Geometry check sheet. Reference: the model listing, model coordinates, mm. Give positions to 0.01 mm unless a question says otherwise; leave off trailing zeros. Write each loop counter-clockwise with the first axis right and the second up, starting at its lowest first coordinate (ties: lowest second). Pieces come first, ordered by that corner, then holes.
(1) Thickness scan on line 1 along X through (y, z) = (8.2, 0); line 2 along Z through (x, y) = (21, 7.75); line 3 along Z through (x, y) = (-41.5, 7.5). Record the ranges inside material, lowest first.
(2) Cross-section at B-B (x = 0). Record the boundary of the cut face in (y, z).
(3) Cross-section at A-A (z = 0). Record the boundary of the cut face in (x, y).
(4) Depth check by flat-ended pin: P1, Ø2, axis at x = 12, y = 8.5, coming from the -Z side; P2, Ø5, axis at y = 1, z = -16, coming from the +X side; P3, Ø3, axis at x = 9, y = 2, coming from the -Z side. Enter the tip coordinate at first touch or a pass-through.
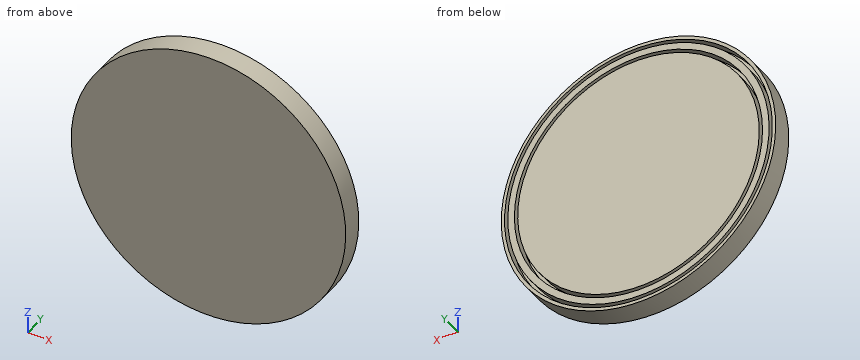
```python
from build123d import *

# Parameters (mm, degrees)
SKETCH2_R           = 62.5
BOSS_EXTRUDE1_DEPTH = 10
SKETCH3_R           = 61
SKETCH3_R_2         = 59.5
SKETCH3_R_3         = 56.5
SKETCH3_R_4         = 55
CUT_EXTRUDE1_DEPTH  = 5


with BuildPart() as part:
    # Sketch2 → Boss-Extrude1 (new body)
    with BuildSketch(Plane(origin=(0, 0, 0), x_dir=(1, 0, 0), z_dir=(0, 1, 0))):
        with Locations(Location((0, 0, 0), (0, 0, 270))):
            Circle(SKETCH2_R)
    extrude(amount=BOSS_EXTRUDE1_DEPTH)

    # Sketch3 → Cut-Extrude1 (cut)
    # profile 1 of 2: a face of its own
    with BuildSketch(Plane(origin=(0, 10, 0), x_dir=(1, 0, 0), z_dir=(0, 1, 0))):
        with Locations(Location((0, 0, 0), (0, 0, 270))):
            Circle(SKETCH3_R)
        with Locations(Location((0, 0, 0), (0, 0, 270))):
            Circle(SKETCH3_R_2, mode=Mode.SUBTRACT)
    # profile 2 of 2: a face of its own
    with BuildSketch(Plane(origin=(0, 10, 0), x_dir=(1, 0, 0), z_dir=(0, 1, 0))):
        with Locations(Location((0, 0, 0), (0, 0, 270))):
            Circle(SKETCH3_R_3)
        with Locations(Location((0, 0, 0), (0, 0, 270))):
            Circle(SKETCH3_R_4, mode=Mode.SUBTRACT)
    extrude(amount=-CUT_EXTRUDE1_DEPTH, mode=Mode.SUBTRACT)


solid = part.part
```
Reply:
1. line 1: x = -62.5 to -61, -59.5 to -56.5, -55 to 55, 56.5 to 59.5, 61 to 62.5
1. line 2: z = -58.87 to -57.27, -55.67 to -52.45, -50.83 to 50.83, 52.45 to 55.67, 57.27 to 58.87
1. line 3: z = -46.73 to -44.71, -42.64 to -38.34, -36.09 to 36.09, 38.34 to 42.64, 44.71 to 46.73
2. outline: (0, -62.5) - (10, -62.5) - (10, -61) - (5, -61) - (5, -59.5) - (10, -59.5) - (10, -56.5) - (5, -56.5) - (5, -55) - (10, -55) - (10, 55) - (5, 55) - (5, 56.5) - (10, 56.5) - (10, 59.5) - (5, 59.5) - (5, 61) - (10, 61) - (10, 62.5) - (0, 62.5) - close
3. outline: (-62.5, 0) - (62.5, 0) - (62.5, 10) - (61, 10) - (61, 5) - (59.5, 5) - (59.5, 10) - (56.5, 10) - (56.5, 5) - (55, 5) - (55, 10) - (-55, 10) - (-55, 5) - (-56.5, 5) - (-56.5, 10) - (-59.5, 10) - (-59.5, 5) - (-61, 5) - (-61, 10) - (-62.5, 10) - close
4. P1: stops at z = -61.52
4. P2: stops at x = 61.02
4. P3: stops at z = -62.05
